from build123d import *

# Parameters (mm, degrees)
CYLINDER_R              = 10
CYLINDER_DEPTH          = 10
CYLINDER001_R           = 2
CYLINDER001_DEPTH       = 30
CYLINDER001_ROLL_ANGLE  = -90
CYLINDER002_R           = 11
CYLINDER002_DEPTH       = 7
CYLINDER002_PITCH_ANGLE = 90
CYLINDER003_R           = 10
CYLINDER003_DEPTH       = 10
CYLINDER003_PITCH_ANGLE = 90
BOX001_W                = 15
BOX001_H                = 10
BOX001_DEPTH            = 15
BOX002_W                = 10
BOX002_H                = 30
BOX002_DEPTH            = 40
BOX_W                   = 40
BOX_H                   = 30
BOX_DEPTH               = 10


with BuildPart() as cylinder:
    # Cylinder → Cylinder (new body)
    with BuildSketch(Plane.XY.offset(-5)):
        Circle(CYLINDER_R)
    extrude(amount=CYLINDER_DEPTH)


with BuildPart() as cylinder001:
    # Cylinder001 → Cylinder001 (new body)
    with BuildSketch(Plane.XY):
        Circle(CYLINDER001_R)
    extrude(amount=CYLINDER001_DEPTH)


with BuildPart() as cylinder001_1:
    # Cylinder001 roll: moved
    add(cylinder001.part.rotate(Axis((0, 0, 0), (1, 0, 0)), CYLINDER001_ROLL_ANGLE))


with BuildPart() as cylinder001_2:
    # Cylinder001 placement: moved
    add(cylinder001_1.part.moved(Location((-15, -15, 0))))


with BuildPart() as bearing_cylinder:
    # Cylinder002 → Cylinder002 (new body)
    with BuildSketch(Plane.XY):
        Circle(CYLINDER002_R)
    extrude(amount=CYLINDER002_DEPTH)


with BuildPart() as bearing_cylinder_1:
    # Cylinder002 pitch: moved
    add(bearing_cylinder.part.rotate(Axis((0, 0, 0), (0, 1, 0)), CYLINDER002_PITCH_ANGLE))


with BuildPart() as bearing_cylinder_2:
    # Cylinder002 placement: moved
    add(bearing_cylinder_1.part.moved(Location((-18.5, 0, 15))))


with BuildPart() as bearing_cylinder_outer:
    # Cylinder003 → Cylinder003 (new body)
    with BuildSketch(Plane.XY):
        Circle(CYLINDER003_R)
    extrude(amount=CYLINDER003_DEPTH)


with BuildPart() as bearing_cylinder_outer_1:
    # Cylinder003 pitch: moved
    add(bearing_cylinder_outer.part.rotate(Axis((0, 0, 0), (0, 1, 0)), CYLINDER003_PITCH_ANGLE))


with BuildPart() as bearing_cylinder_outer_2:
    # Cylinder003 placement: moved
    add(bearing_cylinder_outer_1.part.moved(Location((-20, 0, 15))))


with BuildPart() as negative_fusion:
    # Box001 → Box001 (new body)
    with BuildSketch(Plane(origin=(-20, -5, -5), x_dir=(1, 0, 0), z_dir=(0, 0, 1))):
        with Locations((7.5, 5)):
            Rectangle(BOX001_W, BOX001_H)
    extrude(amount=BOX001_DEPTH)

    # Fusion: union Cylinder, Cylinder001, Bearing Cylinder, Bearing Cylinder Outer
    add(cylinder.part)
    add(cylinder001_2.part)
    add(bearing_cylinder_2.part)
    add(bearing_cylinder_outer_2.part)


with BuildPart() as cube002:
    # Box002 → Box002 (new body)
    with BuildSketch(Plane(origin=(-20, -15, -5), x_dir=(1, 0, 0), z_dir=(0, 0, 1))):
        with Locations((5, 15)):
            Rectangle(BOX002_W, BOX002_H)
    extrude(amount=BOX002_DEPTH)


with BuildPart() as cut:
    # Box → Box (new body)
    with BuildSketch(Plane(origin=(-20, -15, -5), x_dir=(1, 0, 0), z_dir=(0, 0, 1))):
        with Locations((20, 15)):
            Rectangle(BOX_W, BOX_H)
    extrude(amount=BOX_DEPTH)

    # Fusion001: union Cube002
    add(cube002.part)

    # Cut: cut Negative Fusion
    add(negative_fusion.part, mode=Mode.SUBTRACT)


solid = cut.part
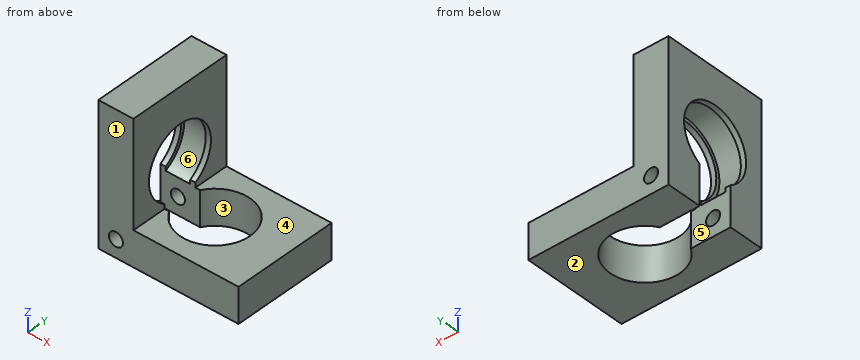
Design review of the part built by this model. Coordinates are the model's own, in mm. Face numbers are marked on the shaded views. A direction names the side the tool comes from. Round coordinates to 2 decimals unless told otherwise and drop trailing zeros. Order: outer loops, then holes, each group sorted by start corner. A loop starts at its lowest first (then second) coordinate and runs counter-clockwise, first axis right, second up. Notation, with made-up numbers: M 3.5,30.25 L 26.5,30.25 A17 cw 26.5,48.25 Z; hole C 82.5,57.5 d2. An arc over 180 degrees is marked long. Answer as CSV lines item,"result". Start each with the question number.
1) Tool access review of the marked faces 4, 5 and 6: name each direction out of +Z, -Z, +X, -X, +Y, -Y from which nothing blocks a thin tool from reaching the whole face with its end or side.
2) Add section B-B (y = -7.5). Give the boundary of the cut face in (x, z).
3) Add section C-C (x = 0). Give the boundary of the cut face in (y, z).
4) Add section D-D (y = 0). Give the boundary of the cut face in (x, z), then the cut area to 3 significant figures.
5) Wall thickness on line 1 along Y through (x, z) = (-9.5, -1); line 2 along X through (y, z) = (8.25, 1.5); line 3 along X through (y, z) = (7.5, 25.5): over which ranges is each line inside the solid? List them lowest first. Write a range as [from, to].
6) Add section A-A (z = 0). Give the boundary of the cut face in (x, y).
7) For pin 1 Ø10.5 at (y, z) = (1.5, 16) entering from +X; pin 2 Ø4.5 at (x, z) = (-15, 0) entering from -Y; pin 3 Ø4 at (y, z) = (6, 22.5) entering from +X; pin 4 Ø3 at (x, y) = (8, 4) entering from +Z, all flat-tipped, find the tip position at first contact; note any pin that passes through.
8) The part is to be moulded in two halves that separate along Y. For the marked faces 1, 2 and 3, say which applies: +Y half, -Y half, draft (parallel to the pull), parting line (faces both ways), or undercut.
Resolved:
1,face 4,"+Z, +X, +Y, -Y"
1,face 5,"-Z, -X"
1,face 6,"none"
2,outline,"M -20,-5 L -6.61,-5 L -6.61,5 L -10,5 L -10,8.39 L -11.5,8.39 L -11.5,6.95 L -18.5,6.95 L -18.5,8.39 L -20,8.39 Z; M -20,21.61 L -18.5,21.61 L -18.5,23.05 L -11.5,23.05 L -11.5,21.61 L -10,21.61 L -10,35 L -20,35 Z; M 6.61,-5 L 20,-5 L 20,5 L 6.61,5 Z; hole C -15,0 d4"
3,outline,"M -15,-5 L -10,-5 L -10,5 L -15,5 Z; M 10,-5 L 15,-5 L 15,5 L 10,5 Z"
4,outline,"M -20,25 L -18.5,25 L -18.5,26 L -11.5,26 L -11.5,25 L -10,25 L -10,35 L -20,35 Z; M 10,-5 L 20,-5 L 20,5 L 10,5 Z"
4,area,"193 mm^2"
5,line 1,"[-15, -5], [5, 15]"
5,line 2,"[-20, -16.32], [-13.68, -5.65], [5.65, 20]"
5,line 3,"[-20, -10]"
6,outline,"M -20,-15 L -17,-15 L -17,-5 L -20,-5 Z; M -20,5 L -17,5 L -17,15 L -20,15 Z; M -13,-15 L 20,-15 L 20,15 L -13,15 L -13,5 L -8.66,5 A10 cw long -8.66,-5 L -13,-5 Z"
7,pin 1,"through"
7,pin 2,"y = -15"
7,pin 3,"x = -10"
7,pin 4,"z = 5"
8,face 1,"-Y half"
8,face 2,"draft"
8,face 3,"undercut"
